from build123d import *

# Parameters (mm, degrees)
T_LE_DE_BASE_PLI_E1_DEPTH = 49.5
ESQUISSE6_R               = 1.75
ENL_V_MAT_EXTRU_1_DEPTH   = 99.371997957
ESQUISSE7_R               = 1.5
ESQUISSE7_W               = 13
ESQUISSE7_H               = 19.5
ESQUISSE7_W_2             = 23
ESQUISSE7_H_2             = 12
ESQUISSE7_W_3             = 15
ESQUISSE7_H_3             = 10
ENL_V_MAT_EXTRU_2_DEPTH   = 1.4
ESQUISSE11_W              = 74
ESQUISSE11_H              = 2
BOSS_EXTRU_2_DEPTH        = 5
CONG_1_R                  = 1


# Sheet-metal steps are written as plain solids
with BuildPart() as part:
    # Esquisse1 → Tôle de base pliée1 (new, symmetric)
    with BuildSketch(Plane(origin=(0, 0, 0), x_dir=(0, 0, -1), z_dir=(1, 0, 0))):
        with BuildLine():
            Line((0, 0), (59.285221502, 0))
            ThreePointArc((59.285221502, 0), (61.671015303, 0.605914437), (63.478574342, 2.276804825))
            Line((63.478574342, 2.276804825), (79.156129603, 26.41812289))
            Line((79.156129603, 26.41812289), (80.330268398, 25.655628241))
            Line((80.330268398, 25.655628241), (64.652713137, 1.514310176))
            ThreePointArc((64.652713137, 1.514310176), (62.339037567, -0.624429521), (59.285221502, -1.4))
            Line((59.285221502, -1.4), (0, -1.4))
            Line((0, -1.4), (0, 0))
        make_face()
    extrude(amount=T_LE_DE_BASE_PLI_E1_DEPTH, both=True)

    # Esquisse6 → Enlèv. mat.-Extru.1 (cut, through all)
    with BuildSketch(Plane.XZ.offset(1.4)):
        with Locations(Location((-43.75, -32, 0), (0, 0, 270))):
            Circle(ESQUISSE6_R)
        with Locations(Location((43.75, -32, 0), (0, 0, 90))):
            Circle(ESQUISSE6_R)
    extrude(amount=-ENL_V_MAT_EXTRU_1_DEPTH, mode=Mode.SUBTRACT)

    # Esquisse7 → Enlèv. mat.-Extru.2 (cut)
    with BuildSketch(Plane.XZ.offset(1.4)):
        with Locations(Location((-28.15, -27, 0), (0, 0, 270))):
            Circle(ESQUISSE7_R)
        with Locations(Location((-4.85, -50.75, 0), (0, 0, 270))):
            Circle(ESQUISSE7_R)
        with Locations(Location((-2.5, -15, 0), (0, 0, 270))):
            Circle(ESQUISSE7_R)
        with Locations(Location((-22.5, -15, 0), (0, 0, 90))):
            Circle(ESQUISSE7_R)
        with Locations((25, -17.75)):
            Rectangle(ESQUISSE7_W, ESQUISSE7_H)
        with Locations((-16.5, -41.75)):
            Rectangle(ESQUISSE7_W_2, ESQUISSE7_H_2)
        with Locations((25, -43.25)):
            Rectangle(ESQUISSE7_W, ESQUISSE7_H)
        with Locations((-12.5, -15)):
            Rectangle(ESQUISSE7_W_3, ESQUISSE7_H_3)
    extrude(amount=-ENL_V_MAT_EXTRU_2_DEPTH, mode=Mode.SUBTRACT)

    # Esquisse11 → Boss.-Extru.2 (add)
    with BuildSketch(Plane(origin=(0, 0, 0), x_dir=(1, 0, 0), z_dir=(0, 1, 0))):
        with Locations((0, 1)):
            Rectangle(ESQUISSE11_W, ESQUISSE11_H)
    extrude(amount=BOSS_EXTRU_2_DEPTH)

    # Congé1
    cong_1_edges = [part.edges().sort_by_distance(p)[0] for p in [
        (-37, 0, -1),
        (37, 0, -1),
        (0, 0, -2),
        (-37, 5, -1),
        (0, 5, 0),
        (37, 5, -1),
        (0, 5, -2),
    ]]
    fillet(cong_1_edges, radius=CONG_1_R - 0.0001)  # a hair under: the kernel refuses the full size


solid = part.part
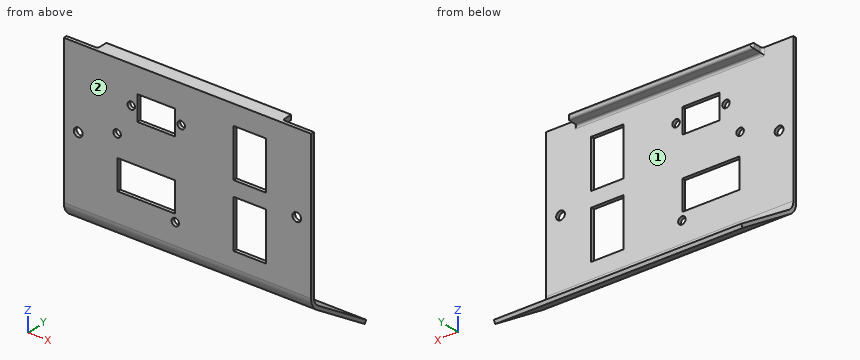
The listing builds one solid part. Answer for the finished solid, in the listing's coordinates (mm). Face numbers are marked on the shaded views. Coordinates: 2 decimals unless noted, no trailing zeros. Loops run counter-clockwise (first coordinate to the right, second up) from the corner with the lowest first, then second, coordinate; pieces in that order, holes last. Notation, with made-up numbers: (-9, 26.25) -> (18, 26.25) arc R20 ccw to (18, 62.25) -> close; hole circle Ø3 at (-39, -3). An arc over 180 degrees is marked (long way). Answer in a Markdown table with one row per item. Add a question column.
1. The part is cut by section B-B, the plane z = -38.5. Write down the section's boundary in (x, y), then the cut area to 3 significant figures.
2. Consider line 1 (X direction, y = -0.7, z = -32); line 2 (X direction, y = -0.85, z = -15); line 3 (X direction, y = -0.45, z = -27). Determine where each line is inside the solid, lowest interval first. Write a range as [from, to].
3. Flat-ended cylindrical pins translate along their axes: P1, Ø1.8, axis at x = -28.15, z = -27, coming from the +Y side; P2, Ø5, axis at x = -4.85, z = -50.75, coming from the +Y side; P3, Ø3, axis at x = -29.5, y = 7.5, coming from the +Z side; P4, Ø1.6, axis at y = 3, z = -1, coming from the -X side. Find the tip coordinate at first contact, or state that the pin passes through.
4. The part is cut by section C-C, the plane x = -43.75. Write down the section's boundary in (y, z).
5. The part is cut by section D-D, the plane z = -15. Write down the section's boundary in (x, y).
6. Determine the mould class of the marked faces 1 and 2 for opening direction Z: +Z half, -Z half, draft (parallel to the pull), parting line (faces both ways), or undercut.
7. The part is cut by section A-A, the plane x = -12. Count the separate pieces of the cut face and the enclosed holes in it, then the cut area to 3 significant figures.
Answer below:
| question | item | result |
|---|---|---|
| 1 | outline | (-49.5, -1.4) -> (-28, -1.4) -> (-28, 0) -> (-49.5, 0) -> close; (-5, -1.4) -> (18.5, -1.4) -> (18.5, 0) -> (-5, 0) -> close; (31.5, -1.4) -> (49.5, -1.4) -> (49.5, 0) -> (31.5, 0) -> close |
| 1 | area | 88.2 mm2 |
| 2 | line 1 | [-49.5, -45.5], [-42, 42], [45.5, 49.5] |
| 2 | line 2 | [-49.5, -24], [-21, -20], [-5, -4], [-1, 18.5], [31.5, 49.5] |
| 2 | line 3 | [-49.5, -29.65], [-26.65, 18.5], [31.5, 49.5] |
| 3 | P1 | through |
| 3 | P2 | y = 0 |
| 3 | P3 | z = -65.9 |
| 3 | P4 | x = -37 |
| 4 | outline | (-1.4, -59.29) arc R6.4 ccw to (1.51, -64.65) -> (25.66, -80.33) -> (26.42, -79.16) -> (2.28, -63.48) arc R5 cw to (0, -59.29) -> (0, -33.75) -> (-1.4, -33.75) -> close; (-1.4, -30.25) -> (0, -30.25) -> (0, 0) -> (-1.4, 0) -> close |
| 5 | outline | (-49.5, -1.4) -> (-24, -1.4) -> (-24, 0) -> (-49.5, 0) -> close; (-21, -1.4) -> (-20, -1.4) -> (-20, 0) -> (-21, 0) -> close; (-5, -1.4) -> (-4, -1.4) -> (-4, 0) -> (-5, 0) -> close; (-1, -1.4) -> (18.5, -1.4) -> (18.5, 0) -> (-1, 0) -> close; (31.5, -1.4) -> (49.5, -1.4) -> (49.5, 0) -> (31.5, 0) -> close |
| 6 | face 1 | undercut |
| 6 | face 2 | draft |
| 7 | separate pieces | 3 |
| 7 | enclosed holes | 0 |
| 7 | area | 110 mm2 |
